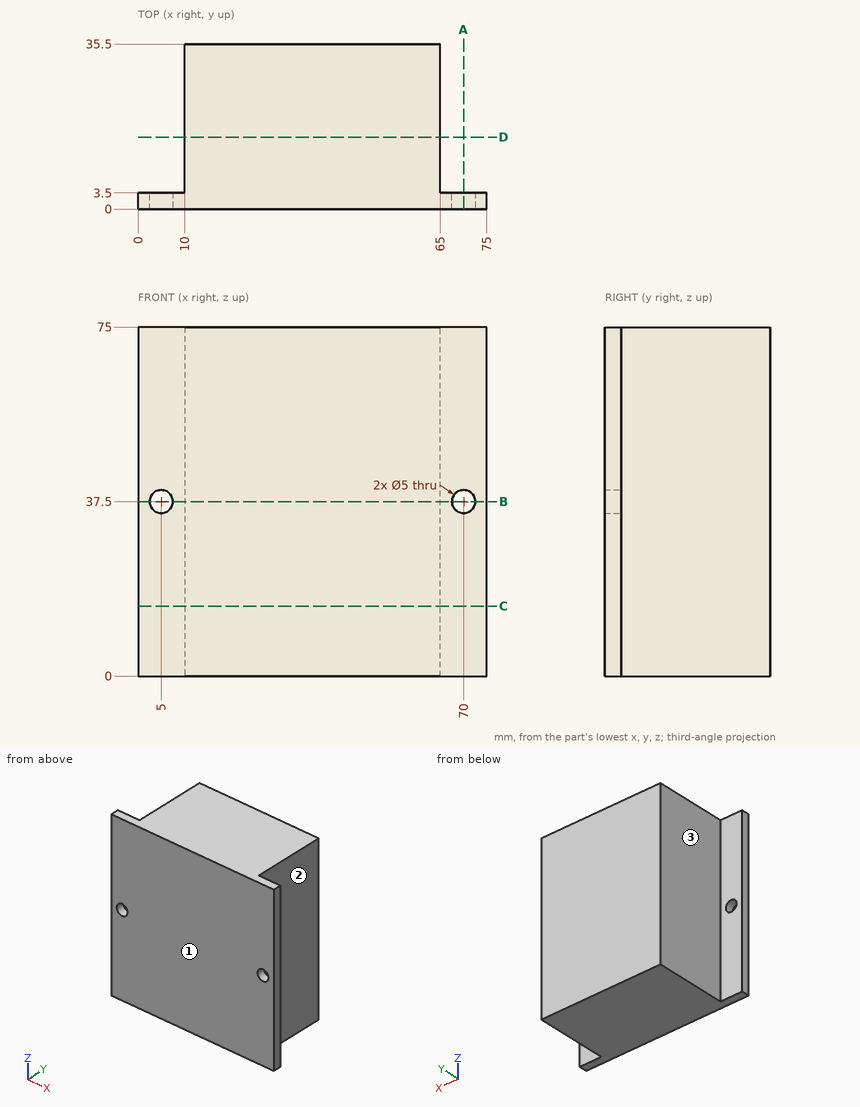
Input: dimensioned drawing with shaded views. Units: mm. Origin: part minimum x, y, z. A direction names the side the tool comes from. Give positions to 0.01 mm unless a question says otherwise; leave off trailing zeros. Loops run counter-clockwise (first coordinate to the right, second up) from the corner with the lowest first, then second, coordinate; pieces in that order, holes last. Notation, with made-up numbers: (65.5, 88.5) - (118.5, 88.5) arc R30 ccw to (118.5, 111.5) - close; hole circle Ø2 at (15.25, 13). An arc over 180 degrees is marked (long way). Answer as CSV lines item,"result". Start each with the question number.
(1) Section query A-A (x = 70). Output: boundary loops of the cut face in (y, z).
(2) Section query D-D (y = 15.5). Output: boundary loops of the cut face in (x, z), and give its area (4 significant figures).
(3) Ray query, line 1 along X through (y, z) = (0.8, 37.5); line 2 along Z through (x, y) = (70, 1); line 3 along X through (y, z) = (7, 41.5). Return the intervals inside material, ascending. Write a range as [from, to].
(4) Section query B-B (z = 37.5). Output: boundary loops of the cut face in (x, y), and give its area (3 significant figures).
(5) Reachability of the marked faces 1, 2 and 3 from +Z, -Z, +X, -X, +Y, -Y: full face, straight path, thin tool, end or side. Return the list, or none.
(6) Section query C-C (z = 15). Output: boundary loops of the cut face in (x, y), and give its area (3 significant figures).
(7) Pin query (flat end, axial travel): P1, Ø8, axis at x = 29, z = 14, coming from the -Y side; P2, Ø6, axis at x = 5, z = 37.5, coming from the +Y side; P3, Ø8, axis at y = 19, z = 10.5, coming from the -X side; P4, Ø10, axis at y = 23, z = 32.5, coming from the +X side. Return the tip coordinate at first contact, or that it passes through.
Worked answers:
1,outline,"(0, 0) - (3.5, 0) - (3.5, 35) - (0, 35) - close; (0, 40) - (3.5, 40) - (3.5, 75) - (0, 75) - close"
2,outline,"(10, 0) - (65, 0) - (65, 75) - (10, 75) - close"
2,area,"4,125 mm^2"
3,line 1,"x = [0, 2.5], [7.5, 67.5], [72.5, 75]"
3,line 2,"z = [0, 35], [40, 75]"
3,line 3,"x = [10, 65]"
4,outline,"(0, 0) - (2.5, 0) - (2.5, 3.5) - (0, 3.5) - close; (7.5, 0) - (67.5, 0) - (67.5, 3.5) - (65, 3.5) - (65, 35.5) - (10, 35.5) - (10, 3.5) - (7.5, 3.5) - close; (72.5, 0) - (75, 0) - (75, 3.5) - (72.5, 3.5) - close"
4,area,"1,990 mm^2"
5,face 1,"+Z, -Z, +X, -X, -Y"
5,face 2,"+Z, -Z, +X, +Y"
5,face 3,"+Z, -Z, -X, +Y"
6,outline,"(0, 0) - (75, 0) - (75, 3.5) - (65, 3.5) - (65, 35.5) - (10, 35.5) - (10, 3.5) - (0, 3.5) - close"
6,area,"2,020 mm^2"
7,P1,"stops at y = 0"
7,P2,"stops at y = 3.5"
7,P3,"stops at x = 10"
7,P4,"stops at x = 65"
